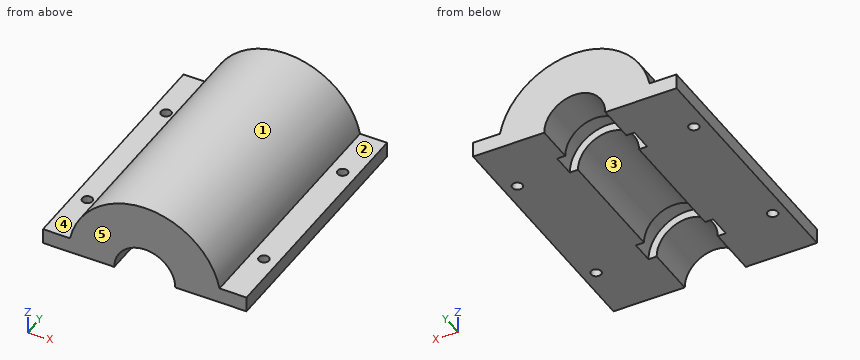
from build123d import *

# Parameters (mm, degrees)
F1_DEPTH = 50
F4_DEPTH = 4.5
F5_START = -28
F5_DEPTH = 4.5
F6_R     = 1
F7_DEPTH = 25


with BuildPart() as f1:
    # F0 (on Front) → F1 (new body)
    with BuildSketch(Plane.XZ):
        with BuildLine():
            Line((0, 3), (0, 0))
            Line((0, 0), (5.0000003353, 0))
            ThreePointArc((5.0000003353, 0), (5.0759580419, 1.5076344304), (5.3030618855, 3))
            Line((5.3030618855, 3), (0, 3))
        make_face()
        with BuildLine():
            ThreePointArc((5.3030618855, 3), (5.0759580419, 1.5076344304), (5.0000003353, 0))
            Line((5.0000003353, 0), (14, 0))
            ThreePointArc((14, 0), (20, 6), (26, 0))
            Line((26, 0), (34.9999996647, 0))
            ThreePointArc((34.9999996647, 0), (34.9240419581, 1.5076344304), (34.6969381145, 3))
            ThreePointArc((34.6969381145, 3), (20, 14.9999996647), (5.3030618855, 3))
        make_face()
        with BuildLine():
            Line((40, 3), (34.6969381145, 3))
            ThreePointArc((34.6969381145, 3), (34.9240419581, 1.5076344304), (34.9999996647, 0))
            Line((34.9999996647, 0), (40, 0))
            Line((40, 0), (40, 3))
        make_face()
    extrude(amount=-F1_DEPTH)

    # F3 (on offset) → F4 (cut)
    with BuildSketch(Plane.XZ.offset(-10)):
        with BuildLine():
            Line((26, 0), (27.6, 0))
            ThreePointArc((27.6, 0), (20, 7.6), (12.4, 0))
            Line((12.4, 0), (14, 0))
            ThreePointArc((14, 0), (20, 6), (26, 0))
        make_face()
    extrude(amount=-F4_DEPTH, mode=Mode.SUBTRACT)

    # F3 (on offset) → F5 (cut)
    with BuildSketch(Plane.XZ.offset(-10).offset(F5_START)):
        with BuildLine():
            Line((26, 0), (27.6, 0))
            ThreePointArc((27.6, 0), (20, 7.6), (12.4, 0))
            Line((12.4, 0), (14, 0))
            ThreePointArc((14, 0), (20, 6), (26, 0))
        make_face()
    extrude(amount=-F5_DEPTH, mode=Mode.SUBTRACT)

    # F6 (on face) → F7 (cut)
    with BuildSketch(Plane.XY.offset(3)):
        with Locations((37.3484690573, 11)):
            Circle(F6_R)
        with Locations((37.3484690573, 39)):
            Circle(F6_R)
        with Locations((2.6515309427, 11)):
            Circle(F6_R)
        with Locations((2.6515309427, 39)):
            Circle(F6_R)
    extrude(amount=-F7_DEPTH, mode=Mode.SUBTRACT)


solid = f1.part
The listing builds one solid part. Answer for the finished solid, in the listing's coordinates (mm). Face numbers are marked on the shaded views. A direction names the side the tool comes from. Give positions to 0.01 mm unless a question says otherwise; leave off trailing zeros. Loops run counter-clockwise (first coordinate to the right, second up) from the corner with the lowest first, then second, coordinate; pieces in that order, holes last.
Item 1: Find the intervals of material crossed by line 1 along Y through (x, z) = (16.5, 6.5); line 2 along Z through (x, y) = (36, 8); line 3 along X through (y, z) = (44, 2.25), in increasing order.
Derived:
line 1: y = 0 to 10, 14.5 to 38, 42.5 to 50
line 2: z = 0 to 3
line 3: x = 0 to 14.44, 25.56 to 40
Item 2: A cutting plane is placed at C-C (x = 20). Give the vertices of the cut face in (y, z).
Derived:
outline: (0, 6) - (10, 6) - (10, 7.6) - (14.5, 7.6) - (14.5, 6) - (38, 6) - (38, 7.6) - (42.5, 7.6) - (42.5, 6) - (50, 6) - (50, 15) - (0, 15) - close
Item 3: A cutting plane is placed at D-D (z = 9). Give the vertices of the cut face in (x, y), then the cut area to 3 significant figures.
Derived:
outline: (8, 0) - (32, 0) - (32, 50) - (8, 50) - close
area: 1,200 mm2
Item 4: Each of these flat-tipped pins is pushed along its axis until it touches: pin 1 Ø1.6 at (x, y) = (37.35, 11) entering from +Z; pin 2 Ø2 at (y, z) = (25.5, 11) entering from -X; pin 3 Ø3 at (y, z) = (15.5, 5.5) entering from -X; pin 4 Ø4 at (x, y) = (1.5, 14.5) entering from +Z. Where does it stop, or does it pass through?
Derived:
pin 1: passes through
pin 2: stops at x = 8.82
pin 3: stops at x = 5.54
pin 4: stops at z = 3
Item 5: Determine the mould class of the marked faces 1, 2 and 3 for opening direction X: +X half, -X half, draft (parallel to the pull), parting line (faces both ways), or undercut.
Derived:
face 1: parting line
face 2: draft
face 3: undercut
Item 6: A cutting plane is placed at B-B (y = 9). Give the vertices of the cut face in (x, z), then the cut area to 3 significant figures.
Derived:
outline: (0, 0) - (14, 0) arc R6 cw to (26, 0) - (40, 0) - (40, 3) - (34.7, 3) arc R15 ccw to (5.3, 3) - (0, 3) - close
area: 327 mm2
Item 7: A cutting plane is placed at A-A (y = 39). Give the vertices of the cut face in (x, z).
Derived:
outline: (0, 0) - (1.65, 0) - (1.65, 3) - (0, 3) - close; (3.65, 0) - (12.4, 0) arc R7.6 cw to (27.6, 0) - (36.35, 0) - (36.35, 3) - (34.7, 3) arc R15 ccw to (5.3, 3) - (3.65, 3) - close; (38.35, 0) - (40, 0) - (40, 3) - (38.35, 3) - close
Item 8: A tool of negligible diameter and unlimited length cuts with its end or side. For the marked faces 4 and 5, from which of +Z, -Z, +X, -X, +Y, -Y can it reach the whole face along a straight path? Write none if from no direction.
Derived:
face 4: +Z, -X, +Y, -Y
face 5: +Z, -Z, +X, -X, -Y
